Verification items for the finished model (mm, model axes). A direction names the side the tool comes from. Round coordinates to 2 decimals unless told otherwise and drop trailing zeros. Use a Markdown table: item, result. Add a question column.
```python
from build123d import *

# Parameters (mm, degrees)
F2_ANGLE  = 180
F1_FACE_R = 21.381984
F3_DEPTH  = 16.256
F4_R      = 13.290294
F5_DEPTH  = 115.57


with BuildPart() as f1:
    # F0 (on Front) → F1 (revolve)
    with BuildSketch(Plane.XZ):
        with BuildLine():
            Line((-44.931725, 21.381984), (-44.931725, 0))
            Line((-44.931725, 0), (0, 0))
            Line((0, 0), (0, 55.869054))
            ThreePointArc((0, 55.869054), (-28.937879, 47.057632), (-44.931725, 21.381984))
        make_face()
    revolve(axis=Axis((-22.465862, 0, 0), (1, 0, 0)))

    # F0 (on Front) → F2 (revolve, symmetric)
    with BuildSketch(Plane.XZ) as f2_sk:
        with BuildLine():
            Line((0, 55.869054), (0, 0))
            Line((0, 0), (56.361724, 0))
            ThreePointArc((56.361724, 0), (41.303803, 41.17319), (0, 55.869054))
        make_face()
    revolve(axis=Axis((28.180862, 0, 0), (1, 0, 0)), revolution_arc=F2_ANGLE / 2)
    revolve(f2_sk.sketch, axis=Axis((28.180862, 0, 0), (-1, 0, 0)), revolution_arc=F2_ANGLE / 2)

    # F1_face (on face) → F3 (join)
    with BuildSketch(Plane(origin=(-44.931725, 0, 0), x_dir=(0, -1, 0), z_dir=(-1, 0, 0))):
        Circle(F1_FACE_R)
    extrude(amount=F3_DEPTH)

    # F4 (on Right) → F5 (cut)
    with BuildSketch(Plane.YZ):
        Circle(F4_R)
    extrude(amount=-F5_DEPTH, mode=Mode.SUBTRACT)


solid = f1.part
```
1) Thickness scan on line 1 (Y direction, x = -17.5, z = 0); line 2 (Z direction, x = -24, y = 0); line 3 (Z direction, x = -41.5, y = 0). Record the ranges inside material, lowest first.
2) Go/stop test with flat-tipped pins: pin 1 (1.5 mm diameter, centred on x = 33, y = 1.5, fed in from -Z); pin 2 (17 mm diameter, centred on y = -1, z = -39, fed in from +X); pin 3 (6.5 mm diameter, centred on y = -0.5, z = 5.5, fed in from -X); pin 4 (1.5 mm diameter, centred on x = -46.5, y = -23, fed in from -Z). Record where each tip stops, or that it passes through.
3) Access from +Z, -Z, +X, -X, +Y, -Y to the whole of each face (thin tool, end or side, straight path). Record for faces 1 (the face through (22, 1, 0)), 2 (the face through (-61.188, -9, 10)).
4) Release check for a two-part mould opening along Z. For faces 3 (the face through (-30.166, 12.677, 3.992)), 4 (the face through (-52.946, 4.635, -20.874)), 5 (the face through (0, -1, -28)), 6 (the face through (0, 0, 5)) record: released by +Z, released by -Z, zero draft, split by the parting line, or undercut.
Geometry results:
| question | item | result |
|---|---|---|
| 1 | line 1 | -53.34 to -13.29, 13.29 to 53.34 |
| 1 | line 2 | -50.33 to -13.29, 13.29 to 50.33 |
| 1 | line 3 | -31.61 to -13.29, 13.29 to 31.61 |
| 2 | pin 1 | z = 0 |
| 2 | pin 2 | x = 0 |
| 2 | pin 3 | x = 0 |
| 2 | pin 4 | through |
| 3 | face 1 | -Z, +X, +Y, -Y |
| 3 | face 2 | +Z, -Z, -X, +Y, -Y |
| 4 | face 3 | undercut |
| 4 | face 4 | split by the parting line |
| 4 | face 5 | zero draft |
| 4 | face 6 | undercut |
